```python
from build123d import *

# Parameters (mm, degrees)
F0_W     = 146.05
F0_H     = 76.2
F0_W_2   = 12.7
F0_H_2   = 63.5
F0_R     = 31.75
F1_DEPTH = 1.5875
F2_SIZE  = 1.5875
F3_SIZE  = 1.5875


with BuildPart() as f1:
    # F0 (on Front) → F1 (new body, symmetric)
    with BuildSketch(Plane.XZ):
        Rectangle(F0_W, F0_H)
        with Locations((-60.861046, 0)):
            Rectangle(F0_W_2, F0_H_2, mode=Mode.SUBTRACT)
        Circle(F0_R, mode=Mode.SUBTRACT)
    extrude(amount=F1_DEPTH, both=True)

    # F2
    f2_edges = [f1.edges().sort_by_distance(p)[0] for p in [
        (-54.511046, -1.5875, 0),
        (-60.861046, -1.5875, -31.75),
        (-67.211046, -1.5875, 0),
        (-60.861046, -1.5875, 31.75),
    ]]
    chamfer(f2_edges, length=F2_SIZE)

    # F3
    f3_edges = [f1.edges().sort_by_distance(p)[0] for p in [
        (-31.75, -1.5875, 0),
    ]]
    chamfer(f3_edges, length=F3_SIZE)


solid = f1.part
```
Work out the finished part from the listing and answer in its coordinate system (mm). Round coordinates to 2 decimals unless told otherwise and drop trailing zeros. Loops run counter-clockwise (first coordinate to the right, second up) from the corner with the lowest first, then second, coordinate; pieces in that order, holes last. Notation, with made-up numbers: M -18.75,-10 L 24.25,-10 A18 cw 24.25,3 Z; hole C 46.25,25 d7. An arc over 180 degrees is marked long. Use CSV: the item, a comma, the result in double quotes.
Q1. Section A-A, the plane x = 0 is taken. Determine the outline of the cut face in (y, z), then the cut area to 3 significant figures.
Determined:
outline,"M -1.59,-38.1 L 1.59,-38.1 L 1.59,-31.75 L 0,-31.75 L -1.59,-33.34 Z; M -1.59,33.34 L 0,31.75 L 1.59,31.75 L 1.59,38.1 L -1.59,38.1 Z"
area,"37.8 mm2"
Q2. Section C-C, the plane z = 0 is taken. State how many separate pieces and enclosed holes the cut face has, then the cut area to 3 significant figures.
Determined:
separate pieces,"3"
enclosed holes,"0"
area,"217 mm2"
Q3. The mould has two halves that part along Z. Classify faces 1 (the flat face through (-1, 0, -38.1)), 2 (the cylindrical face through (-6.883, 0.805, -30.995)), 3 (the flat face through (-73.025, 0, -1)): pulls with the +Z half, pulls with the -Z half, needs draft (parallel to the pull), parting line crosses it, or undercut.
Determined:
face 1,"pulls with the -Z half"
face 2,"undercut"
face 3,"needs draft"
Q4. Consider L1, parallel to Z at x = 0, y = 0.65; L2, parallel to X at y = -0.4, z = -20.5 (3 decimals); L3, parallel to X at y = -1.15, z = 0.5 (3 decimals). Determine where each line is inside the solid, lowest interval first.
Determined:
L1,"-38.1 to -31.75, 31.75 to 38.1"
L2,"-73.025 to -67.611, -54.111 to -24.766, 24.766 to 73.025"
L3,"-73.025 to -68.361, -53.361 to -32.896, 32.896 to 73.025"
Q5. Section B-B, the plane y = 0.95 is taken. Determine the outline of the cut face in (x, z) (3 decimals).
Determined:
outline,"M -73.025,-38.1 L 73.025,-38.1 L 73.025,38.1 L -73.025,38.1 Z; hole M -67.211,-31.75 L -54.511,-31.75 L -54.511,31.75 L -67.211,31.75 Z; hole C 0,0 d63.5"
